Model file for the job. Use its own axes, mm. A direction names the side the tool comes from. Round coordinates to 2 decimals unless told otherwise and drop trailing zeros. Order: outer loops, then holes, each group sorted by start corner. A loop starts at its lowest first (then second) coordinate and runs counter-clockwise, first axis right, second up. Notation, with made-up numbers: (-25.75, -33.5) - (1.25, -33.5) arc R31 cw to (1.25, -4.5) - close; hole circle Ø4 at (68.5, 12). An arc over 180 degrees is marked (long way). Use one line per item in the form item = value.
from build123d import *

# Parameters (mm, degrees)
PAD_DEPTH            = 6.5
POCKET_DEPTH         = 6
SKETCH002_R          = 13.5
POCKET001_DEPTH      = 1
SKETCH003_W          = 5.4
SKETCH003_H          = 6.5
PAD001_DEPTH         = 3.5
POCKET002_DEPTH      = 10
SKETCH010_W          = 3.95
SKETCH010_H          = 6.5
PAD002_DEPTH         = 3.5
POCKET005_DEPTH      = 10
SKETCH014_R          = 20.45
SKETCH014_R_2        = 19.85
POCKET008_DEPTH      = 0.3
SKETCH015_R          = 2.2
SKETCH015_R_2        = 0.975
PAD003_DEPTH         = 2
POCKET009_DEPTH      = 4
POCKET010_DEPTH      = 4
PAD004_DEPTH         = 4
POCKET013_DEPTH      = 12.151
POCKET013_DEPTH_BACK = 36.251
SKETCH022_R          = 0.6
POCKET014_DEPTH      = 2
SKETCH023_R          = 0.6
POCKET015_DEPTH      = 2


with BuildPart() as part:
    # Sketch → Pad (new body)
    with BuildSketch(Plane.XY):
        with BuildLine():
            Line((-22.5019915649, 16), (-22.5019915649, -16))
            Line((-22.5019915649, -16), (-16.2858834578, -17.9))
            ThreePointArc((-16.2858834578, -17.9), (-0.4552796053, -24.1957169863), (15.6009615088, -18.5))
            Line((15.6009615088, -18.5), (24.5395016581, -17.45))
            Line((24.5395016581, 17.45), (24.5395016581, -17.45))
            Line((15.6009615088, 18.5), (24.5395016581, 17.45))
            ThreePointArc((15.6009615088, 18.5), (-0.4552796053, 24.1957169863), (-16.2858834578, 17.9))
            Line((-22.5019915649, 16), (-16.2858834578, 17.9))
        make_face()
    extrude(amount=PAD_DEPTH)

    # Sketch001 → Pocket (cut)
    with BuildSketch(Plane.XY):
        with BuildLine():
            Line((-14.8539557021, 16.9), (-21.2122180433, 15.55))
            Line((-21.2122180433, 15.55), (-21.2122180433, -15.55))
            Line((-21.2122180433, -15.55), (-14.8539557021, -16.9))
            ThreePointArc((-14.8539557021, -16.9), (-0.0760301383, -22.4998715423), (14.739402973, -17))
            Line((14.739402973, -17), (23.6191552218, -16.4))
            Line((23.6191552218, 16.4), (23.6191552218, -16.4))
            Line((14.739402973, 17), (23.6191552218, 16.4))
            ThreePointArc((14.739402973, 17), (-0.0760301383, 22.4998715423), (-14.8539557021, 16.9))
        make_face()
    extrude(amount=POCKET_DEPTH, mode=Mode.SUBTRACT)

    # Sketch002 (on Face19 of Pocket) → Pocket001 (cut)
    with BuildSketch(Plane(origin=(0, 0, 6), x_dir=(1, 0, 0), z_dir=(0, 0, -1))):
        Circle(SKETCH002_R)
    extrude(amount=-POCKET001_DEPTH, mode=Mode.SUBTRACT)

    # Sketch003 (on Face7 of Pad) → Pad001 (join)
    with BuildSketch(Plane.YZ.offset(24.5395016581)):
        with Locations((-14.75, 3.25)):
            Rectangle(SKETCH003_W, SKETCH003_H)
        with Locations((14.75, 3.25)):
            Rectangle(SKETCH003_W, SKETCH003_H)
    extrude(amount=PAD001_DEPTH)

    # Sketch006 (on Face22 of Pad001) → Pocket002 (cut)
    with BuildSketch(Plane.XY.offset(6.5)):
        with BuildLine():
            ThreePointArc((24.5395016581, 17.45), (26.1592830786, 16.2095505764), (28.0395016581, 15.4176006311))
            Line((28.0395016581, 17.45), (28.0395016581, 15.4176006311))
            Line((28.0395016581, 17.45), (24.5395016581, 17.45))
        make_face()
        with BuildLine():
            ThreePointArc((28.0395016581, -15.4176006311), (26.1592830786, -16.2095505765), (24.5395016581, -17.4500000001))
            Line((28.0395016581, -17.45), (24.5395016581, -17.45))
            Line((28.0395016581, -15.4176006311), (28.0395016581, -17.45))
        make_face()
    extrude(amount=-POCKET002_DEPTH, mode=Mode.SUBTRACT)

    # Sketch010 (on Face3 of Pad) → Pad002 (join)
    with BuildSketch(Plane(origin=(-22.5019915649, 0, 0), x_dir=(0, -1, 0), z_dir=(-1, 0, 0))):
        with Locations((-14.025, 3.25)):
            Rectangle(SKETCH010_W, SKETCH010_H)
        with Locations((14.025, 3.25)):
            Rectangle(SKETCH010_W, SKETCH010_H)
    extrude(amount=PAD002_DEPTH)

    # Sketch011 (on Face28 of Pad002) → Pocket005 (cut)
    with BuildSketch(Plane.XY.offset(6.5)):
        Polygon((-26.0019915649, 16), (-22.5019915649, 16), (-26.0019915649, 14.5), align=None)
        Polygon((-22.5019915649, -16), (-26.0019915649, -14.5), (-26.0019915649, -16), align=None)
    extrude(amount=-POCKET005_DEPTH, mode=Mode.SUBTRACT)

    # Sketch014 (on Face10 of Pad) → Pocket008 (cut)
    with BuildSketch(Plane.XY.offset(6.5)):
        Circle(SKETCH014_R)
        Circle(SKETCH014_R_2, mode=Mode.SUBTRACT)
    extrude(amount=-POCKET008_DEPTH, mode=Mode.SUBTRACT)

    # Sketch015 (on Face19 of Pocket) → Pad003 (join)
    with BuildSketch(Plane(origin=(0, 0, 6), x_dir=(1, 0, 0), z_dir=(0, 0, -1))):
        with Locations((-18.42, 13.32)):
            Circle(SKETCH015_R)
        with Locations((-18.42, 13.32)):
            Circle(SKETCH015_R_2, mode=Mode.SUBTRACT)
        with Locations((7.27, 18.56)):
            Circle(SKETCH015_R)
        with Locations((7.27, 18.56)):
            Circle(SKETCH015_R_2, mode=Mode.SUBTRACT)
        with Locations((5.37, -19.79)):
            Circle(SKETCH015_R)
        with Locations((5.37, -19.79)):
            Circle(SKETCH015_R_2, mode=Mode.SUBTRACT)
        with Locations((-18.42, -13.32)):
            Circle(SKETCH015_R)
        with Locations((-18.42, -13.32)):
            Circle(SKETCH015_R_2, mode=Mode.SUBTRACT)
    extrude(amount=PAD003_DEPTH)

    # Sketch016 (on Face4 of Pocket) → Pocket009 (cut)
    with BuildSketch(Plane(origin=(0, 0, 0), x_dir=(1, 0, 0), z_dir=(0, 0, -1))):
        with BuildLine():
            Line((-4.9992330338, 23.6779996848), (-5.0007669662, 21.9372361465))
            ThreePointArc((5.0007669662, 21.9372361465), (0, 22.5), (-5.0007669662, 21.9372361465))
            Line((5.0007669662, 23.6776757675), (5.0007669662, 21.9372361465))
            ThreePointArc((5.0007669662, 23.6776757675), (0.00078388, 24.1999999873), (-4.9992330338, 23.6779996848))
        make_face()
    extrude(amount=-POCKET009_DEPTH, mode=Mode.SUBTRACT)

    # Sketch017 (on Face4 of Pocket) → Pocket010 (cut)
    with BuildSketch(Plane(origin=(0, 0, 0), x_dir=(1, 0, 0), z_dir=(0, 0, -1))):
        with BuildLine():
            ThreePointArc((-3.2541322314, -22.2634369184), (0, -22.5), (3.2541322314, -22.2634369184))
            Line((3.2541322314, -22.2634369184), (3.5, -23.9455632634))
            ThreePointArc((-3.5, -23.9455632634), (0, -24.2), (3.5, -23.9455632634))
            Line((-3.2541322314, -22.2634369184), (-3.5, -23.9455632634))
        make_face()
        with BuildLine():
            ThreePointArc((-13.9498796389, -17.6536358312), (-11.25, -19.4855715851), (-8.3135572795, -20.9077680626))
            Line((-8.3135572795, -20.9077680626), (-8.9416927184, -22.487466094))
            ThreePointArc((-15.0038705449, -18.987466094), (-12.1, -20.9578147716), (-8.9416927184, -22.487466094))
            Line((-13.9498796389, -17.6536358312), (-15.0038705449, -18.987466094))
        make_face()
        with BuildLine():
            ThreePointArc((8.3135572795, -20.9077680626), (11.25, -19.4855715851), (13.9498796389, -17.6536358312))
            Line((13.9498796389, -17.6536358312), (15.0038705449, -18.987466094))
            ThreePointArc((8.9416927184, -22.487466094), (12.1, -20.9578147716), (15.0038705449, -18.987466094))
            Line((8.3135572795, -20.9077680626), (8.9416927184, -22.487466094))
        make_face()
    extrude(amount=-POCKET010_DEPTH, mode=Mode.SUBTRACT)

    # Sketch018 (on Face8 of Pocket005) → Pad004 (join)
    with BuildSketch(Plane(origin=(0, 0, 0), x_dir=(1, 0, 0), z_dir=(0, 0, -1))):
        Polygon((-26.0019915649, 14.5), (-26.0019915649, 12.05), (-22.5019915649, 12.05), (-22.5019915649, 16), align=None)
        Polygon((-26.0019915649, -12.05), (-22.5019915649, -12.05), (-22.5019915649, -16), (-26.0019915649, -14.5), align=None)
        with BuildLine():
            Line((24.5395016581, 17.4500000001), (24.5395016581, 12.05))
            Line((28.0395016581, 12.05), (24.5395016581, 12.05))
            Line((28.0395016581, 15.4176006311), (28.0395016581, 12.05))
            ThreePointArc((24.5395016581, 17.4500000001), (26.1592830786, 16.2095505765), (28.0395016581, 15.4176006311))
        make_face()
        with BuildLine():
            Line((24.5395016581, -12.05), (24.5395016581, -17.45))
            ThreePointArc((28.0395016581, -15.4176006311), (26.1592830786, -16.2095505764), (24.5395016581, -17.45))
            Line((28.0395016581, -12.05), (28.0395016581, -15.4176006311))
            Line((24.5395016581, -12.05), (28.0395016581, -12.05))
        make_face()
    extrude(amount=PAD004_DEPTH)

    # Sketch021 (on Face50 of Pad004) → Pocket013 (cut, two sides)
    with BuildSketch(Plane(origin=(0, -12.05, 0), x_dir=(-1, 0, 0), z_dir=(0, 1, 0))) as pocket013_sk:
        with BuildLine():
            Line((-24.8620157143, 6.5), (-28.0395016581, 6.5))
            Line((-28.0395016581, 6.5), (-28.0395016581, 2.1))
            ThreePointArc((-24.8620157143, 6.5), (-26.8441838951, 4.5841143344), (-28.0395016581, 2.1))
        make_face()
        with BuildLine():
            ThreePointArc((-25.9995016581, -4), (-25.0260575173, -3.5134441408), (-24.5395016581, -2.54))
            Line((-24.5395016581, -4), (-24.5395016581, -2.54))
            Line((-24.5395016581, -4), (-25.9995016581, -4))
        make_face()
        with BuildLine():
            Line((22.5019915649, -4), (22.5019915649, -2.54))
            ThreePointArc((22.5019915649, -2.54), (22.9885474241, -3.5134441408), (23.9619915649, -4))
            Line((22.5019915649, -4), (23.9619915649, -4))
        make_face()
        with BuildLine():
            Line((26.0019915649, 6.5), (26.0019915649, 2.1))
            ThreePointArc((26.0019915649, 2.1), (24.806673802, 4.5841143344), (22.8245056212, 6.5))
            Line((26.0019915649, 6.5), (22.8245056212, 6.5))
        make_face()
    extrude(amount=-POCKET013_DEPTH, mode=Mode.SUBTRACT)
    extrude(pocket013_sk.sketch, amount=POCKET013_DEPTH_BACK, mode=Mode.SUBTRACT)

    # Sketch022 (on Face66 of Pocket013) → Pocket014 (cut)
    with BuildSketch(Plane.XZ.offset(-12.05)):
        with Locations((-24.7019915649, -2.7)):
            Circle(SKETCH022_R)
        with Locations((26.7395016581, -2.7)):
            Circle(SKETCH022_R)
    extrude(amount=-POCKET014_DEPTH, mode=Mode.SUBTRACT)

    # Sketch023 (on Face49 of Pocket014) → Pocket015 (cut)
    with BuildSketch(Plane(origin=(0, -12.05, 0), x_dir=(-1, 0, 0), z_dir=(0, 1, 0))):
        with Locations((-26.7395016581, -2.7)):
            Circle(SKETCH023_R)
        with Locations((24.7019915649, -2.7)):
            Circle(SKETCH023_R)
    extrude(amount=-POCKET015_DEPTH, mode=Mode.SUBTRACT)


solid = part.part
(1) Slice it at B-B on y = 0. Give the cut face in (x, z), then the cut area to 3 significant figures.
Report:
outline = (-22.5, 0) - (-21.21, 0) - (-21.21, 6) - (-13.5, 6) - (-13.5, 6.5) - (-19.85, 6.5) - (-19.85, 6.2) - (-20.45, 6.2) - (-20.45, 6.5) - (-22.5, 6.5) - close; (13.5, 6) - (23.62, 6) - (23.62, 0) - (24.54, 0) - (24.54, 6.5) - (20.45, 6.5) - (20.45, 6.2) - (19.85, 6.2) - (19.85, 6.5) - (13.5, 6.5) - close
area = 22.9 mm2
(2) Tool access for faces 1 (the face through (26, 12.05, 1)), 2 (the face through (-0.2, 24.2, 4.6)), 3 (the face through (19.117, 16.704, 2.958)), 4 (the face through (-24.1, -13, -2.7)), 5 (the face through (-24, 12.05, 1)): list every direction of +Z, -Z, +X, -X, +Y, -Y with a clear straight run to the whole face (end or side of a thin tool).
Report:
face_1 = +Z, -Z, +X
face_2 = +Z, -Z, +Y
face_3 = -Z
face_4 = none
face_5 = +Z, -Z, -X
(3) Probe probe 1 along Y at (x, z) = (0, 6.4); probe 2 along X at (y, z) = (-14.5, 5.25); probe 3 along X at (y, z) = (-7, 1). List the from-to ranges inside material, lowest first. Write a range as [from, to].
Report:
probe_1 = [-24.2, -20.45], [-19.85, -13.5], [13.5, 19.85], [20.45, 24.2]
probe_2 = [-24.27, -21.21], [-20.28, -16.56], [23.62, 26.31]
probe_3 = [-22.5, -21.21], [23.62, 24.54]
(4) Slice it at C-C on z = 1. Count the separate pieces of the cut face and the enclosed holes in it, then the cut area to 3 significant figures.
Report:
separate_pieces = 4
enclosed_holes = 0
area = 224 mm2
(5) Pin check, flat tips, straight feed: pin 1 (2.5 mm diameter, centred on x = 5.5, y = 22, fed in from -Z); pin 2 (3 mm diameter, centred on x = 15, z = 3, fed in from +Y); pin 3 (1.5 mm diameter, centred on y = 2, z = 4, fed in from +X). Stop position of each tip, or through.
Report:
pin_1 = 0
pin_2 = 19.82
pin_3 = 24.54
(6) Slice it at A-A on x = 0. Give the cut face in (y, z), then the cut area to 3 significant figures.
Report:
outline = (-24.2, 4) - (-22.5, 4) - (-22.5, 6) - (-13.5, 6) - (-13.5, 6.5) - (-19.85, 6.5) - (-19.85, 6.2) - (-20.45, 6.2) - (-20.45, 6.5) - (-24.2, 6.5) - close; (13.5, 6) - (22.5, 6) - (22.5, 4) - (24.2, 4) - (24.2, 6.5) - (20.45, 6.5) - (20.45, 6.2) - (19.85, 6.2) - (19.85, 6.5) - (13.5, 6.5) - close
area = 17.1 mm2
(7) Pull direction Z, two halves, no side cores. Call faces 6 (the face through (-25, 14.05, -3)), 7 (the face through (26.82, 14, 4.62)), 8 (the face through (27, 14, -4)), 9 (the face through (27, -14.05, -3)): released by +Z, released by -Z, zero draft, split by the parting line, or undercut.
Report:
face_6 = undercut
face_7 = released by +Z
face_8 = released by -Z
face_9 = undercut
